Geometry: final body of the model. Coordinates: model frame, mm. Face numbers are marked on the shaded views. A direction names the side the tool comes from. Give positions to 0.01 mm unless a question says otherwise; leave off trailing zeros. Order: outer loops, then holes, each group sorted by start corner. A loop starts at its lowest first (then second) coordinate and runs counter-clockwise, first axis right, second up. Notation, with made-up numbers: (-29, -3.5) -> (29, -3.5) arc R11 cw to (29, 4.5) -> close; hole circle Ø2 at (21.25, 56.25). An arc over 180 degrees is marked (long way). Answer in a Markdown table with one row per item. Add a question column.
Q1. Cut plane C-C on y = 0. Return the cut outline in (x, z).
Q2. Contact query for flat-ended pins moving along their axis: P1, Ø3.5, axis at x = -25.5, z = 2, coming from the -Y side; P2, Ø4, axis at y = 24, z = 3.5, coming from the -X side; P3, Ø3, axis at x = 31.5, z = 4, coming from the -Y side; P4, Ø13, axis at x = 0, y = 0, coming from the -Z side. Output: stop coordinate, or through.
Q3. Cut plane D-D on z = 4.5. Count the separate pieces of the cut face and the enclosed holes in it, and give its area (3 significant figures).
Q4. Line query: line 1 along Y through (x, z) = (0, 3) (3 decimals); line 2 along X through (y, z) = (-17, 6.25); line 3 along Y through (x, z) = (-20, 0.5). Output: solid intervals per line, ascending. Write a range as from..to.
Q5. Cut plane B-B on y = 38. Return the cut outline in (x, z), and give its area (3 significant figures).
Q6. Cut plane A-A on x = 0. Return the cut outline in (y, z) (3 decimals).
Q7. Pull-direction query (Y, two-part tool) for the marked faces 3, 4 and 5; classes: +Y half, -Y half, draft (parallel to the pull), parting line (faces both ways), or undercut.
Q8. Set-up query: the marked faces 1 and 2. Return all of +Z, -Z, +X, -X, +Y, -Y with unobstructed straight access to the full face (end or side cutting, diameter ignored); none if empty.
from build123d import *

# Parameters (mm, degrees)
F0_R     = 11
F1_DEPTH = 7
F3_DEPTH = 31


with BuildPart() as f1:
    # F0 (on Top) → F1 (new body)
    with BuildSketch(Plane.XY):
        with BuildLine():
            ThreePointArc((-35.690819, -5.735916), (-38.971143, -22.5), (-22.812859, -28.041198))
            ThreePointArc((-22.812859, -28.041198), (-17.02025, -23.393855), (-14.717093, -16.333573))
            ThreePointArc((-14.717093, -16.333573), (-14.713883, -16.1668), (-14.712813, -16))
            ThreePointArc((-14.712813, -16), (-16.538809, -9.356082), (-21.503836, -4.57859))
            ThreePointArc((-21.503836, -4.57859), (-28.769798, -3.043041), (-35.690819, -5.735916))
        make_face()
        with BuildLine():
            ThreePointArc((-13.875123, -1.865735), (-13.961542, 1.036992), (-13.447237, 3.8951))
            ThreePointArc((-13.447237, 3.8951), (-26.298738, 3.074491), (-35.690819, -5.735916))
            ThreePointArc((-35.690819, -5.735916), (-28.769798, -3.043041), (-21.503836, -4.57859))
            ThreePointArc((-21.503836, -4.57859), (-18.141279, -1.951674), (-13.875123, -1.865735))
        make_face()
        with BuildLine():
            ThreePointArc((-22.812859, -28.041198), (-10.486782, -24.312621), (-3.350363, -13.593199))
            ThreePointArc((-3.350363, -13.593199), (-6.08271, -12.609546), (-8.553336, -11.083341))
            ThreePointArc((-8.553336, -11.083341), (-10.760839, -14.734971), (-14.717093, -16.333573))
            ThreePointArc((-14.717093, -16.333573), (-17.02025, -23.393855), (-22.812859, -28.041198))
        make_face()
        with BuildLine():
            ThreePointArc((13.875123, -1.865735), (13.968746, -0.934955), (14, 0))
            ThreePointArc((14, 0), (13.861121, 1.967063), (13.447237, 3.8951))
            ThreePointArc((13.447237, 3.8951), (12.124356, 7), (10.096874, 9.698099))
            ThreePointArc((10.096874, 9.698099), (7.878832, 11.572554), (5.321787, 12.949076))
            ThreePointArc((5.321787, 12.949076), (0, 14), (-5.321787, 12.949076))
            ThreePointArc((-5.321787, 12.949076), (-7.878832, 11.572554), (-10.096874, 9.698099))
            ThreePointArc((-10.096874, 9.698099), (-12.124356, 7), (-13.447237, 3.8951))
            ThreePointArc((-13.447237, 3.8951), (-13.961542, 1.036992), (-13.875123, -1.865735))
            ThreePointArc((-13.875123, -1.865735), (-12.124356, -7), (-8.553336, -11.083341))
            ThreePointArc((-8.553336, -11.083341), (-6.08271, -12.609546), (-3.350363, -13.593199))
            ThreePointArc((-3.350363, -13.593199), (0, -14), (3.350363, -13.593199))
            ThreePointArc((3.350363, -13.593199), (6.08271, -12.609546), (8.553336, -11.083341))
            ThreePointArc((8.553336, -11.083341), (12.124356, -7), (13.875123, -1.865735))
        make_face()
        Circle(F0_R, mode=Mode.SUBTRACT)
        with BuildLine():
            ThreePointArc((-10.096874, 9.698099), (-7.878832, 11.572554), (-5.321787, 12.949076))
            ThreePointArc((-5.321787, 12.949076), (-7.38044, 16.686646), (-6.786742, 20.912163))
            ThreePointArc((-6.786742, 20.912163), (-11.749548, 26.436896), (-12.87796, 33.777114))
            ThreePointArc((-12.87796, 33.777114), (-15.811956, 21.23813), (-10.096874, 9.698099))
        make_face()
        with BuildLine():
            ThreePointArc((13, 32), (12.969454, 32.89065), (12.87796, 33.777114))
            ThreePointArc((12.87796, 33.777114), (0, 45), (-12.87796, 33.777114))
            ThreePointArc((-12.87796, 33.777114), (-11.749548, 26.436896), (-6.786742, 20.912163))
            ThreePointArc((-6.786742, 20.912163), (0, 19), (6.786742, 20.912163))
            ThreePointArc((6.786742, 20.912163), (11.340804, 25.644988), (13, 32))
        make_face()
        with BuildLine():
            ThreePointArc((5.321787, 12.949076), (7.878832, 11.572554), (10.096874, 9.698099))
            ThreePointArc((10.096874, 9.698099), (15.811956, 21.23813), (12.87796, 33.777114))
            ThreePointArc((12.87796, 33.777114), (12.969454, 32.89065), (13, 32))
            ThreePointArc((13, 32), (11.340804, 25.644988), (6.786742, 20.912163))
            ThreePointArc((6.786742, 20.912163), (7.38044, 16.686646), (5.321787, 12.949076))
        make_face()
        with BuildLine():
            ThreePointArc((13.447237, 3.8951), (13.861121, 1.967063), (14, 0))
            ThreePointArc((14, 0), (13.968746, -0.934955), (13.875123, -1.865735))
            ThreePointArc((13.875123, -1.865735), (18.141279, -1.951674), (21.503836, -4.57859))
            ThreePointArc((21.503836, -4.57859), (28.769798, -3.043041), (35.690819, -5.735916))
            ThreePointArc((35.690819, -5.735916), (26.298738, 3.074491), (13.447237, 3.8951))
        make_face()
        with BuildLine():
            ThreePointArc((14.717093, -16.333573), (10.760839, -14.734971), (8.553336, -11.083341))
            ThreePointArc((8.553336, -11.083341), (6.08271, -12.609546), (3.350363, -13.593199))
            ThreePointArc((3.350363, -13.593199), (10.486782, -24.312621), (22.812859, -28.041198))
            ThreePointArc((22.812859, -28.041198), (17.02025, -23.393855), (14.717093, -16.333573))
        make_face()
        with BuildLine():
            ThreePointArc((40.712813, -16), (39.390015, -10.286598), (35.690819, -5.735916))
            ThreePointArc((35.690819, -5.735916), (28.769798, -3.043041), (21.503836, -4.57859))
            ThreePointArc((21.503836, -4.57859), (16.454483, -9.5), (14.717093, -16.333573))
            ThreePointArc((14.717093, -16.333573), (17.02025, -23.393855), (22.812859, -28.041198))
            ThreePointArc((22.812859, -28.041198), (34.968866, -26.786552), (40.712813, -16))
        make_face()
    extrude(amount=F1_DEPTH)

    # F2 (on face) → F3 (cut)
    with BuildSketch(Plane.XY.offset(7)):
        Polygon((-38.584318, -16), (-33.148566, -25.415), (-22.27706, -25.415), (-16.841307, -16), (-22.27706, -6.585), (-33.148566, -6.585), align=None)
        Polygon((33.148566, -25.415), (38.584318, -16), (33.148566, -6.585), (22.27706, -6.585), (16.841307, -16), (22.27706, -25.415), align=None)
        Polygon((5.435753, 41.415), (-5.435753, 41.415), (-10.871506, 32), (-5.435753, 22.585), (5.435753, 22.585), (10.871506, 32), align=None)
    extrude(amount=-F3_DEPTH, mode=Mode.SUBTRACT)


solid = f1.part
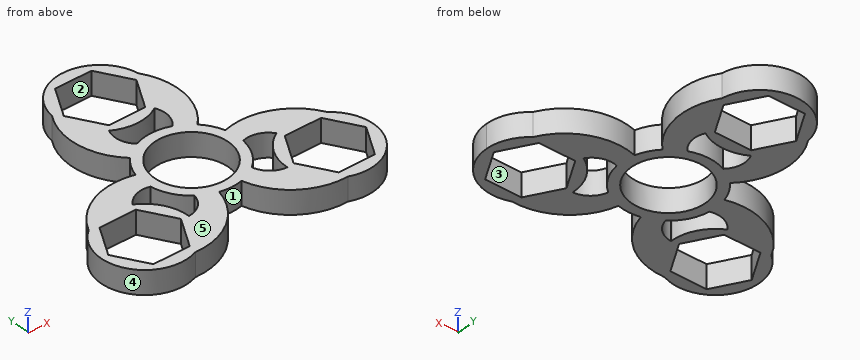
Completed:
| question | item | result |
|---|---|---|
| 1 | outline | (-31.19, 0) -> (-11, 0) -> (-11, 7) -> (-31.19, 7) -> close; (11, 0) -> (31.19, 0) -> (31.19, 7) -> (11, 7) -> close |
| 2 | P1 | stops at y = -28.99 |
| 2 | P2 | stops at x = -15.94 |
| 2 | P3 | stops at y = -28.8 |
| 2 | P4 | passes through |
| 3 | separate pieces | 1 |
| 3 | enclosed holes | 7 |
| 3 | area | 1,630 mm² |
| 4 | line 1 | y = -14..-11, 11..14, 19..22.585, 41.415..45 |
| 4 | line 2 | x = -40.67..-38.01, -17.42..-4.55, 4.55..17.42, 38.01..40.67 |
| 4 | line 3 | y = -27.98..-21.47, -10.53..-5.54, -2.96..4.6 |
| 5 | outline | (-11.53, 0) -> (-7.41, 0) -> (-7.41, 7) -> (-11.53, 7) -> close; (7.41, 0) -> (11.53, 0) -> (11.53, 7) -> (7.41, 7) -> close |
| 5 | area | 57.8 mm² |
| 6 | outline | (-14, 0) -> (-11, 0) -> (-11, 7) -> (-14, 7) -> close; (11, 0) -> (14, 0) -> (14, 7) -> (11, 7) -> close; (19, 0) -> (22.585, 0) -> (22.585, 7) -> (19, 7) -> close; (41.415, 0) -> (45, 0) -> (45, 7) -> (41.415, 7) -> close |
| 7 | face 3 | undercut |
| 7 | face 4 | parting line |
| 7 | face 5 | draft |
| 8 | face 1 | +Z, -Z, -Y |
| 8 | face 2 | +Z, -Z |
